```python
from build123d import *

# Parameters (mm, degrees)
SKETCH_1_W          = 40
SKETCH_1_H          = 20
EXTRUDE_1_DEPTH     = 40.45
EXTRUDE_2_DEPTH     = 3
FILLET_1_R          = 2
SKETCH_4_W          = 40
SKETCH_4_H          = 20
SKETCH_4_W_2        = 39
SKETCH_4_H_2        = 19
CUT_EXTRUDE_2_DEPTH = 0.5
SKETCH_5_W          = 40
SKETCH_5_H          = 20
SKETCH_5_W_2        = 39
SKETCH_5_H_2        = 19
CUT_EXTRUDE_3_DEPTH = 0.5
SKETCH_6_R          = 6
EXTRUDE_3_DEPTH     = 1
FILLET_2_R          = 1
SKETCH_7_R          = 5
SKETCH_7_R_2        = 3
SKETCH_7_R_3        = 2.5
CUT_EXTRUDE_4_DEPTH = 0.5
CUT_EXTRUDE_6_DEPTH = 1
CUT_EXTRUDE_7_DEPTH = 1
CUT_EXTRUDE_8_DEPTH = 54.103963207
EXTRUDE_START       = 5
SKETCH_11_R         = 2.5
EXTRUDE_4_DEPTH     = 5
SKETCH_12_R         = 1.5
CUT_EXTRUDE_9_DEPTH = 0.5
FILLET_3_R          = 0.5


with BuildPart() as part:
    # 草图1 → 凸台-拉伸1 (new body)
    with BuildSketch(Plane(origin=(0, 0, 0), x_dir=(1, 0, 0), z_dir=(0, 1, 0))):
        Rectangle(SKETCH_1_W, SKETCH_1_H)
    extrude(amount=EXTRUDE_1_DEPTH)

    # 草图2 → 凸台-拉伸2 (add)
    with BuildSketch(Plane(origin=(0, 27.65, 0), x_dir=(-1, 0, 0), z_dir=(0, -1, 0))):
        with BuildLine():
            Line((20, 9.2), (27.22, 9.2))
            Line((27.22, 9.2), (27.22, 5.65))
            Line((27.22, 5.65), (25.599038106, 5.65))
            ThreePointArc((25.599038106, 5.65), (22.8, 4.9), (25.599038106, 4.15))
            Line((25.599038106, 4.15), (27.22, 4.15))
            Line((27.22, 4.15), (27.22, -4.15))
            Line((27.22, -4.15), (25.599038106, -4.15))
            ThreePointArc((25.599038106, -4.15), (22.8, -4.9), (25.599038106, -5.65))
            Line((25.599038106, -5.65), (27.22, -5.65))
            Line((27.22, -5.65), (27.22, -9.2))
            Line((27.22, -9.2), (20, -9.2))
            Line((20, -9.2), (20, 9.2))
        make_face()
        with BuildLine():
            Line((-20, 9.2), (-20, -9.2))
            Line((-20, -9.2), (-27.22, -9.2))
            Line((-27.22, -9.2), (-27.22, -5.65))
            Line((-27.22, -5.65), (-25.599038106, -5.65))
            ThreePointArc((-25.599038106, -5.65), (-22.8, -4.9), (-25.599038106, -4.15))
            Line((-25.599038106, -4.15), (-27.22, -4.15))
            Line((-27.22, -4.15), (-27.22, 4.15))
            Line((-27.22, 4.15), (-25.599038106, 4.15))
            ThreePointArc((-25.599038106, 4.15), (-22.8, 4.9), (-25.599038106, 5.65))
            Line((-25.599038106, 5.65), (-27.22, 5.65))
            Line((-27.22, 5.65), (-27.22, 9.2))
            Line((-27.22, 9.2), (-20, 9.2))
        make_face()
    extrude(amount=-EXTRUDE_2_DEPTH)

    # 圆角1
    fillet_1_edges = [part.edges().sort_by_distance(p)[0] for p in [
        (-27.22, 29.15, -9.2),
        (-27.22, 29.15, 9.2),
        (27.22, 29.15, -9.2),
        (27.22, 29.15, 9.2),
    ]]
    fillet(fillet_1_edges, radius=FILLET_1_R)

    # 草图4 → 切除-拉伸2 (cut)
    with BuildSketch(Plane(origin=(0, 27.65, 0), x_dir=(-1, 0, 0), z_dir=(0, -1, 0))):
        Rectangle(SKETCH_4_W, SKETCH_4_H)
        Rectangle(SKETCH_4_W_2, SKETCH_4_H_2, mode=Mode.SUBTRACT)
    extrude(amount=CUT_EXTRUDE_2_DEPTH, mode=Mode.SUBTRACT)

    # 草图5 → 切除-拉伸3 (cut)
    with BuildSketch(Plane(origin=(0, 10, 0), x_dir=(-1, 0, 0), z_dir=(0, -1, 0))):
        Rectangle(SKETCH_5_W, SKETCH_5_H)
        Rectangle(SKETCH_5_W_2, SKETCH_5_H_2, mode=Mode.SUBTRACT)
    extrude(amount=CUT_EXTRUDE_3_DEPTH, mode=Mode.SUBTRACT)

    # 草图6 → 凸台-拉伸3 (add)
    with BuildSketch(Plane(origin=(0, 40.45, 0), x_dir=(1, 0, 0), z_dir=(0, 1, 0))):
        with Locations(Location((-10, 0, 0), (0, 0, 90))):
            Circle(SKETCH_6_R)
    extrude(amount=EXTRUDE_3_DEPTH)

    # 圆角2
    fillet_2_edges = [part.edges().sort_by_distance(p)[0] for p in [
        (-10, 41.45, 6),
    ]]
    fillet(fillet_2_edges, radius=FILLET_2_R - 0.0001)  # a hair under: the kernel refuses the full size

    # 草图7 → 切除-拉伸4 (cut)
    # profile 1 of 6: a face of its own
    with BuildSketch(Plane(origin=(0, 41.45, 0), x_dir=(1, 0, 0), z_dir=(0, 1, 0))):
        with Locations((-10, 0)):
            Circle(SKETCH_7_R)
        with Locations(Location((-10, 0, 0), (0, 0, 270))):
            Circle(SKETCH_7_R_2, mode=Mode.SUBTRACT)
    # profile 2 of 6: a face of its own
    with BuildSketch(Plane(origin=(0, 41.45, 0), x_dir=(1, 0, 0), z_dir=(0, 1, 0))):
        with BuildLine():
            Line((-14.943429983, 0.75), (-15.3, 0.75))
            Line((-15.3, 0.75), (-15.3, -0.75))
            Line((-15.3, -0.75), (-14.943429983, -0.75))
            ThreePointArc((-14.943429983, -0.75), (-15, 0), (-14.943429983, 0.75))
        make_face()
    # profile 3 of 6: a face of its own
    with BuildSketch(Plane(origin=(0, 41.45, 0), x_dir=(1, 0, 0), z_dir=(0, 1, 0))):
        with BuildLine():
            ThreePointArc((-9.25, -4.943429983), (-10, -5), (-10.75, -4.943429983))
            Line((-10.75, -4.943429983), (-10.75, -5.3))
            Line((-10.75, -5.3), (-9.25, -5.3))
            Line((-9.25, -5.3), (-9.25, -4.943429983))
        make_face()
    # profile 4 of 6: a face of its own
    with BuildSketch(Plane(origin=(0, 41.45, 0), x_dir=(1, 0, 0), z_dir=(0, 1, 0))):
        with BuildLine():
            Line((-4.7, 0.75), (-5.056570017, 0.75))
            ThreePointArc((-5.056570017, 0.75), (-5.014162562, 0.376065209), (-5, 0))
            ThreePointArc((-5, 0), (-5.014162562, -0.376065209), (-5.056570017, -0.75))
            Line((-5.056570017, -0.75), (-4.7, -0.75))
            Line((-4.7, -0.75), (-4.7, 0.75))
        make_face()
    # profile 5 of 6: a face of its own
    with BuildSketch(Plane(origin=(0, 41.45, 0), x_dir=(1, 0, 0), z_dir=(0, 1, 0))):
        with BuildLine():
            Line((-10.75, 5.3), (-10.75, 4.943429983))
            ThreePointArc((-10.75, 4.943429983), (-10, 5), (-9.25, 4.943429983))
            Line((-9.25, 4.943429983), (-9.25, 5.3))
            Line((-9.25, 5.3), (-10.75, 5.3))
        make_face()
    # profile 6 of 6: a face of its own
    with BuildSketch(Plane(origin=(0, 41.45, 0), x_dir=(1, 0, 0), z_dir=(0, 1, 0))):
        with Locations(Location((-10, 0, 0), (0, 0, 270))):
            Circle(SKETCH_7_R_3)
    extrude(amount=-CUT_EXTRUDE_4_DEPTH, mode=Mode.SUBTRACT)

    # 草图8 → 切除-拉伸6 (cut)
    with BuildSketch(Plane(origin=(0, 40.45, 0), x_dir=(1, 0, 0), z_dir=(0, 1, 0))):
        with BuildLine():
            Line((-10, 9), (20, 9))
            Line((20, 9), (20, 10))
            Line((20, 10), (-20, 10))
            Line((-20, 10), (-20, -10))
            Line((-20, -10), (20, -10))
            Line((20, -10), (20, -9))
            Line((20, -9), (-10, -9))
            ThreePointArc((-10, -9), (-19, 0), (-10, 9))
        make_face()
    extrude(amount=-CUT_EXTRUDE_6_DEPTH, mode=Mode.SUBTRACT)

    # 草图9 → 切除-拉伸7 (cut)
    with BuildSketch(Plane.XY.offset(10)):
        Polygon((6, 39.45), (20, 34.95), (20, 39.45), align=None)
    cut_extrude_7 = extrude(amount=-CUT_EXTRUDE_7_DEPTH, mode=Mode.SUBTRACT)

    # 镜向1: 切除-拉伸7 across plane
    add(cut_extrude_7.mirror(Plane.XY), mode=Mode.SUBTRACT)

    # 草图10 → 切除-拉伸8 (cut, through all)
    with BuildSketch(Plane.XY.offset(9)):
        Polygon((14, 40.45), (16.4, 36.107142857), (20, 34.95), (20, 40.45), align=None)
    extrude(amount=-CUT_EXTRUDE_8_DEPTH, mode=Mode.SUBTRACT)

    # 草图11 → 凸台-拉伸4 (add)
    with BuildSketch(Plane(origin=(0, 40.95, 0), x_dir=(1, 0, 0), z_dir=(0, 1, 0)).offset(EXTRUDE_START)):
        with Locations(Location((-10, 0, 0), (0, 0, 270))):
            Circle(SKETCH_11_R)
    extrude(amount=-EXTRUDE_4_DEPTH)

    # 草图12 → 切除-拉伸9 (cut)
    with BuildSketch(Plane(origin=(0, 45.95, 0), x_dir=(1, 0, 0), z_dir=(0, 1, 0))):
        with Locations(Location((-10, 0, 0), (0, 0, 270))):
            Circle(SKETCH_12_R)
    extrude(amount=-CUT_EXTRUDE_9_DEPTH, mode=Mode.SUBTRACT)

    # 圆角3
    fillet_3_edges = [part.edges().sort_by_distance(p)[0] for p in [
        (-10, 45.95, -2.5),
    ]]
    fillet(fillet_3_edges, radius=FILLET_3_R)


solid = part.part
```
Design review of the part built by this model. Coordinates are the model's own, in mm. A direction names the side the tool comes from. Coordinates: 2 decimals unless noted, no trailing zeros. Order: outer loops, then holes, each group sorted by start corner. A loop starts at its lowest first (then second) coordinate and runs counter-clockwise, first axis right, second up. Notation, with made-up numbers: (88, -19) - (144, -19) arc R24 ccw to (144, 2) - close; hole circle Ø9 at (56.25, 76). An arc over 180 degrees is marked (long way). Answer in a Markdown table with one row per item.
(1) For faces 1 (the flat face through (6, 40, -9)), 2 (the flat face through (-19, 39.45, -3)), 3 (the cylindrical face through (-12.44, 43.48, -0.54)), 4 (the flat face through (-20, 18, 0)), 5 (the flat face through (24, 30.65, 0)), list the 3-axis set-ups (+Z, -Z, +X, -X, +Y, -Y) from which the entire face can be reached by the end or side of a thin tool; tool diameter is ignored.
Checked values:
| item | result |
|---|---|
| face 1 | -Z, +X, +Y |
| face 2 | -X, +Y |
| face 3 | +Y |
| face 4 | +Z, -Z, -X, -Y |
| face 5 | +Z, -Z, +X, +Y |
(2) Consider section C-C on y = 43.5. State the section outline as (x, z) points, plus the area to 3 significant figures.
Checked values:
| item | result |
|---|---|
| outline | circle Ø5 at (-10, 0) |
| area | 19.6 mm^2 |
(3) The part is to be moulded in two halves that separate along X. For faces 6 (the flat face through (0.1, 10, -9.7)), 7 (the flat face through (27.22, 29, 0)), 8 (the cylindrical face through (-7.026, 41.204, -0.391)), say which applies: released by +X, released by -X, zero draft, split by the parting line, or undercut.
Checked values:
| item | result |
|---|---|
| face 6 | zero draft |
| face 7 | released by +X |
| face 8 | undercut |
(4) Wall thickness on line 1 along Z through (x, y) = (-24.3, 29.2); line 2 along X through (y, z) = (29.9, 4.9); line 3 along X through (y, z) = (3, -8): over which ranges is each line inside the solid? List them lowest first. Write a range as from..to.
Checked values:
| item | result |
|---|---|
| line 1 | -9.2..-6.4, -3.4..3.4, 6.4..9.2 |
| line 2 | -22.8..22.8 |
| line 3 | -20..20 |
(5) Clearance check with flat-ended pins moving along their axes: pin 1 (0.5 mm diameter, centred on x = -26.5, y = 29, fed in from -Z); pin 2 (3.5 mm diameter, centred on x = -23, z = -3, fed in from +Y); pin 3 (1.3 mm diameter, centred on x = 26.5, y = 29.5, fed in from +Z). State where each tip first meets the part, or that it passes through.
Checked values:
| item | result |
|---|---|
| pin 1 | z = -8.91 |
| pin 2 | y = 30.65 |
| pin 3 | z = 9.1 |
(6) Consider section D-D on y = 20.5. State the section outline as (x, z) points, plus the area to 3 significant figures.
Checked values:
| item | result |
|---|---|
| outline | (-20, -10) - (20, -10) - (20, 10) - (-20, 10) - close |
| area | 800 mm^2 |
(7) Consider section B-B on x = 4.5. State the section outline as (y, z) points, plus the area to 3 significant figures.
Checked values:
| item | result |
|---|---|
| outline | (0, -10) - (9.5, -10) - (9.5, -9.5) - (10, -9.5) - (10, -10) - (27.15, -10) - (27.15, -9.5) - (27.65, -9.5) - (27.65, -10) - (39.45, -10) - (39.45, -9) - (40.45, -9) - (40.45, 9) - (39.45, 9) - (39.45, 10) - (27.65, 10) - (27.65, 9.5) - (27.15, 9.5) - (27.15, 10) - (10, 10) - (10, 9.5) - (9.5, 9.5) - (9.5, 10) - (0, 10) - close |
| area | 806 mm^2 |
(8) Consider section A-A on x = 24.3. State the section outline as (y, z) points, plus the area to 3 significant figures.
Checked values:
| item | result |
|---|---|
| outline | (27.65, -9.2) - (30.65, -9.2) - (30.65, -6.4) - (27.65, -6.4) - close; (27.65, -3.4) - (30.65, -3.4) - (30.65, 3.4) - (27.65, 3.4) - close; (27.65, 6.4) - (30.65, 6.4) - (30.65, 9.2) - (27.65, 9.2) - close |
| area | 37.2 mm^2 |
